Can you work these out from the model? Positions are in its coordinate system, mm. A direction names the side the tool comes from. Coordinates: 2 decimals unless noted, no trailing zeros. Loops run counter-clockwise (first coordinate to the right, second up) from the corner with the lowest first, then second, coordinate; pieces in that order, holes last.
```python
from build123d import *

# Parameters (mm, degrees)
BOSS_EXTRUDE1_DEPTH     = 0.798558565
SKETCH2_W               = 5.08
SKETCH2_H               = 10.16
BOSS_EXTRUDE3_DEPTH     = 1.27
MIRROR2_COPY_1_SKETCH_W = 5.08
MIRROR2_COPY_1_SKETCH_H = 10.16
MIRROR2_COPY_1_DEPTH    = 1.27
SKETCH3_R               = 1.27
CUT_EXTRUDE1_DEPTH      = 5.13711713


with BuildPart() as part:
    # Sketch1 → Boss-Extrude1 (new body, symmetric)
    with BuildSketch(Plane.XY):
        with BuildLine():
            Line((-25.4, 0), (-15.113, 0))
            ThreePointArc((-15.113, 0), (0, 15.113), (15.113, 0))
            Line((15.113, 0), (25.4, 0))
            Line((25.4, 0), (25.4, 21.463))
            Line((25.4, 21.463), (-25.4, 21.463))
            Line((-25.4, 21.463), (-25.4, 0))
        make_face()
    extrude(amount=BOSS_EXTRUDE1_DEPTH, both=True)

    # Sketch2 → Boss-Extrude3 (add)
    with BuildSketch(Plane.XY.offset(0.798558565)):
        with Locations((22.86, 5.08)):
            Rectangle(SKETCH2_W, SKETCH2_H)
        with Locations((22.86, -5.08)):
            Rectangle(SKETCH2_W, SKETCH2_H)
    boss_extrude3 = extrude(amount=BOSS_EXTRUDE3_DEPTH)

    # Mirror1: Boss-Extrude3 across plane
    add(boss_extrude3.mirror(Plane.XY))

    # Mirror2: Boss-Extrude3 across plane
    add(boss_extrude3.mirror(Plane(origin=(0, 0, 0), x_dir=(0, 0, 1), z_dir=(1, 0, 0))))

    # Mirror2 copy 1 sketch → Mirror2 copy 1 (add)
    with BuildSketch(Plane(origin=(0, 0, -0.798558565), x_dir=(-1, 0, 0), z_dir=(0, 0, -1))):
        with Locations((22.86, 5.08)):
            Rectangle(MIRROR2_COPY_1_SKETCH_W, MIRROR2_COPY_1_SKETCH_H)
        with Locations((22.86, -5.08)):
            Rectangle(MIRROR2_COPY_1_SKETCH_W, MIRROR2_COPY_1_SKETCH_H)
    extrude(amount=MIRROR2_COPY_1_DEPTH)

    # Sketch3 → Cut-Extrude1 (cut, through all)
    with BuildSketch(Plane(origin=(0, 0, -2.068558565), x_dir=(-1, 0, 0), z_dir=(0, 0, -1))):
        with Locations((-22.86, -5.334)):
            Circle(SKETCH3_R)
    cut_extrude1 = extrude(amount=-CUT_EXTRUDE1_DEPTH, mode=Mode.SUBTRACT)

    # Mirror3: Cut-Extrude1 across plane
    add(cut_extrude1.mirror(Plane(origin=(0, 0, 0), x_dir=(0, 0, 1), z_dir=(1, 0, 0))), mode=Mode.SUBTRACT)


solid = part.part
```
(1) I'm going to push flat-ended pins straight in: pin 1 (1.8 mm diameter, centred on x = 22, z = 0, fed in from -Y); pin 2 (10 mm diameter, centred on x = 2.5, y = 12.5, fed in from +Z); pin 3 (1 mm diameter, centred on x = -23.5, z = -1.5, fed in from +Y); pin 4 (10.5 mm diameter, centred on x = -7.5, y = 6.5, fed in from -Z). Where does each tip first touch, or does it pass through?
Check values:
pin 1: stops at y = -10.16
pin 2: stops at z = 0.8
pin 3: stops at y = 10.16
pin 4: stops at z = -0.8
(2) Which directions (+Z, -Z, +X, -X, +Y, -Y) give clear straight access to the entire face, cutting with the end or side of a thin tool? Please do faces 1 (the flat face through (-23, 10.16, 1)), 2 (the flat face through (22.8, -3.9, 0.799)), 3 (the flat face through (20.32, 0, -1)), 4 (the flat face through (20.32, 0, 1)), 5 (the flat face through (23, 0, 2.069)).
Check values:
face 1: +Z, +X, -X, +Y
face 2: +X, -X, -Y
face 3: -Z, +Y, -Y
face 4: +Z, +Y, -Y
face 5: +Z, +X, -X, +Y, -Y
(3) I want a section at B-B on x = -22.86. Write out the boundary of the cut face in (y, z), then the cut area to 3 significant figures.
Check values:
outline: (-10.16, -2.07) - (-6.6, -2.07) - (-6.6, -0.8) - (-10.16, -0.8) - close; (-10.16, 0.8) - (-6.6, 0.8) - (-6.6, 2.07) - (-10.16, 2.07) - close; (-4.06, -2.07) - (10.16, -2.07) - (10.16, -0.8) - (21.46, -0.8) - (21.46, 0.8) - (10.16, 0.8) - (10.16, 2.07) - (-4.06, 2.07) - (-4.06, 0.8) - (0, 0.8) - (0, -0.8) - (-4.06, -0.8) - close
area: 79.4 mm2
(4) I want a section at D-D on x = 0. Write out the boundary of the cut face in (y, z), then the cut area to 3 significant figures.
Check values:
outline: (15.11, -0.8) - (21.46, -0.8) - (21.46, 0.8) - (15.11, 0.8) - close
area: 10.1 mm2
(5) If we mould it in two halves opening along Z, with no side actions, what happens to faces 6 (the flat face through (-22.8, -3.9, 0.799)), 7 (the flat face through (23, 0, -2.069)), 8 (the flat face through (25.4, 2, 0))? For each: released by +Z, released by -Z, zero draft, split by the parting line, or undercut.
Check values:
face 6: undercut
face 7: released by -Z
face 8: zero draft
(6) I want a section at A-A on y = -0.5. Write out the boundary of the cut face in (x, z).
Check values:
outline: (-25.4, -2.07) - (-20.32, -2.07) - (-20.32, -0.8) - (-25.4, -0.8) - close; (-25.4, 0.8) - (-20.32, 0.8) - (-20.32, 2.07) - (-25.4, 2.07) - close; (20.32, -2.07) - (25.4, -2.07) - (25.4, -0.8) - (20.32, -0.8) - close; (20.32, 0.8) - (25.4, 0.8) - (25.4, 2.07) - (20.32, 2.07) - close
(7) If I drill on probe 1 along Y at (x, z) = (22.86, -1.3); probe 2 along X at (y, z) = (-4, 0.9); probe 3 along X at (y, z) = (-5, 1.25), over which ranges is the centre line in solid material (lowest first)?
Check values:
probe 1: y = -10.16 to -6.6, -4.06 to 10.16
probe 2: x = -25.4 to -20.32, 20.32 to 25.4
probe 3: x = -25.4 to -24.09, -21.63 to -20.32, 20.32 to 21.63, 24.09 to 25.4
(8) I want a section at C-C on y = 5. Write out the boundary of the cut face in (x, z).
Check values:
outline: (-25.4, -2.07) - (-20.32, -2.07) - (-20.32, -0.8) - (-14.26, -0.8) - (-14.26, 0.8) - (-20.32, 0.8) - (-20.32, 2.07) - (-25.4, 2.07) - close; (14.26, -0.8) - (20.32, -0.8) - (20.32, -2.07) - (25.4, -2.07) - (25.4, 2.07) - (20.32, 2.07) - (20.32, 0.8) - (14.26, 0.8) - close
